Can you work these out from the model? Positions are in its coordinate system, mm. A direction names the side the tool comes from. Coordinates: 2 decimals unless noted, no trailing zeros. Loops run counter-clockwise (first coordinate to the right, second up) from the corner with the lowest first, then second, coordinate; pieces in that order, holes last. Notation, with made-up numbers: (-8, 79) -> (-2, 79) arc R23 ccw to (-2, 100) -> close; hole circle Ø7 at (37, -30). An arc over 180 degrees is marked (long way). Use one line per item in the form item = value. Start each with the question number.
(1) Imagine slicing it at D-D (x = -9.25). List the corners of the cut face in (y, z) for me.
(2) Imagine slicing it at C-C (z = -5.5). List the corners of the cut face in (x, y) for me.
(3) Imagine slicing it at A-A (y = 0). List the corners of the cut face in (x, z) for me.
(4) Thinking about a two-plate mould opening in Y: for faces 1 (the cylindrical face through (-2.17, -9.76, 0.49)), 2 (the flat face through (-5, 9, 1)), which applies, released by +Y, released by -Y, zero draft, split by the parting line, or undercut?
(5) I need wall thicknesses on line 1 (Y direction, x = 0, z = -1.5); line 2 (Y direction, x = 0, z = 0.6); line 3 (Z direction, x = 7, y = -5). Which ranges of each line are inside material? Lowest first, please. Write a range as [from, to].
(6) I'm going to push flat-ended pins straight in: pin 1 (3 mm diameter, centred on x = 2.5, y = -0.5, fed in from +Z); pin 2 (2 mm diameter, centred on x = -9.5, z = 0, fed in from -Y); pin 3 (2 mm diameter, centred on x = 6.5, z = 0, fed in from -Y); pin 4 (6 mm diameter, centred on x = 1.5, y = 9, fed in from +Z). Where does each tip first touch, or does it pass through?
(7) On a 3-axis mill with a long thin cutter (end or side, diameter ignored), from which of +Z, -Z, +X, -X, +Y, -Y can I reach the whole of each face in a straight line? I mean faces 3 (the flat face through (-4.3, 0.1, 0)), 4 (the flat face through (3, 3, -6)). Say none if no direction works.
```python
from build123d import *

# Parameters (mm, degrees)
SKETCH1_R           = 12
SKETCH1_R_2         = 10
BOSS_EXTRUDE1_DEPTH = 1
BOSS_EXTRUDE2_START = 6
SKETCH2_R           = 12
BOSS_EXTRUDE2_DEPTH = 6
SKETCH3_R           = 4
CUT_EXTRUDE1_DEPTH  = 13


with BuildPart() as part:
    # Sketch1 → Boss-Extrude1 (new body)
    with BuildSketch(Plane(origin=(0, 0, 0), x_dir=(0, 1, 0), z_dir=(0, 0, 1))):
        with Locations(Location((0, 0, 0), (0, 0, 270))):
            Circle(SKETCH1_R)
        with Locations(Location((0, 0, 0), (0, 0, 270))):
            Circle(SKETCH1_R_2, mode=Mode.SUBTRACT)
    extrude(amount=BOSS_EXTRUDE1_DEPTH)

    # Sketch2 → Boss-Extrude2 (add)
    with BuildSketch(Plane(origin=(0, 0, 0), x_dir=(1, 0, 0), z_dir=(0, 0, -1)).offset(BOSS_EXTRUDE2_START)):
        with Locations(Location((0, 0, 0), (0, 0, 180))):
            Circle(SKETCH2_R)
    extrude(amount=-BOSS_EXTRUDE2_DEPTH)

    # Sketch3 → Cut-Extrude1 (cut)
    with BuildSketch(Plane.XY):
        Circle(SKETCH3_R)
    extrude(amount=-CUT_EXTRUDE1_DEPTH, mode=Mode.SUBTRACT)


solid = part.part
```
Worked out:
q1.outline = (-7.64, -6) -> (7.64, -6) -> (7.64, 1) -> (3.8, 1) -> (3.8, 0) -> (-3.8, 0) -> (-3.8, 1) -> (-7.64, 1) -> close
q2.outline = circle Ø24 at (0, 0); hole circle Ø8 at (0, 0)
q3.outline = (-12, -6) -> (-4, -6) -> (-4, 0) -> (-10, 0) -> (-10, 1) -> (-12, 1) -> close; (4, -6) -> (12, -6) -> (12, 1) -> (10, 1) -> (10, 0) -> (4, 0) -> close
q4.face_1 = undercut
q4.face_2 = zero draft
q5.line_1 = [-12, -4], [4, 12]
q5.line_2 = [-12, -10], [10, 12]
q5.line_3 = [-6, 0]
q6.pin_1 = 0
q6.pin_2 = -8.47
q6.pin_3 = -10.67
q6.pin_4 = 1
q7.face_3 = +Z
q7.face_4 = -Z, +X, -X, +Y, -Y
